from build123d import *

# Parameters (mm, degrees)
F1_DEPTH = 2.54
F4_D     = 6.7564
F5_R     = 5.08
F6_R     = 5.08
F9_D     = 3
F10_D    = 3


with BuildPart() as f1:
    # F0 (on Top) → F1 (new body)
    with BuildSketch(Plane.XY):
        Polygon((-26.9663626849, 16.0324431312), (-26.6666630804, 3.3142461729), (-10.6108812243, 3.3142461729), (-10.6108812243, -5.1539645243), (-26.3746562004, -5.1539645243), (-26.6666630804, -16.9342223267), (-10.6108812243, -17.3322101165), (9.2456126958, -17.3322101165), (9.2456126958, 11.2262545153), (65.6030206382, 11.518263258), (65.6030206382, 16.1625675214), (-11.1902779489, 16.1625675214), align=None)
    extrude(amount=F1_DEPTH)


with BuildPart() as f1_1:
    # F2: moved
    add(f1.part.moved(Location((-33.782, 26.162, 0))))

    # F4 (through all)
    with Locations(Plane.XY.offset(2.54)):
        with Locations((-35.1868793368, 26.1346530169)):
            Hole(F4_D / 2)

    # F5
    f5_edges = [f1_1.edges().sort_by_distance(p)[0] for p in [
        (-60.448663, 9.227778, 1.27),
    ]]
    fillet(f5_edges, radius=F5_R)

    # F6
    f6_edges = [f1_1.edges().sort_by_distance(p)[0] for p in [
        (-60.748363, 42.194443, 1.27),
    ]]
    fillet(f6_edges, radius=F6_R)

    # F9 (through all)
    with Locations(Plane.XY.offset(2.54)):
        with Locations((-52.7054518143, 42.2607827135)):
            Hole(F9_D / 2)

    # F10 (through all)
    with Locations(Plane.XY.offset(2.54)):
        with Locations((-52.9959336795, 9.0430407773)):
            Hole(F10_D / 2)


solid = f1_1.part
Part model, mm, in its own coordinate system. A direction names the side the tool comes from. Coordinates: 2 decimals unless noted, no trailing zeros. Loops run counter-clockwise (first coordinate to the right, second up) from the corner with the lowest first, then second, coordinate; pieces in that order, holes last. Notation, with made-up numbers: (12.25, 4) - (23.25, 4) arc R22 ccw to (23.25, 25) - close; hole circle Ø10 at (-21.5, 87.5). An arc over 180 degrees is marked (long way). Write each question's results on one line, items separated by ' | '. Start each with the question number.
Q1. Which spindle directions (+Z, -Z, +X, -X, +Y, -Y) get a long thin tool onto all of the face, cutting with end or side? Do faces 4 (the flat face through (-6, 42.325, 1)), 5 (the flat face through (-24.536, 23, 1)), 6 (the flat face through (-53, 29.476, 1)). Say none if no direction does.
Q2. Slice it at C-C on y = 11.5. Give the cut face in (x, z), and give its area (3 significant figures).
Q3. Slice it at A-A on z = 1.7. Give the cut face in (x, y), and give its area (3 significant figures).
Q4. Two-plate mould, pull along Y, no slides. Class faces 1 (the flat face through (-44.393, 25, 1)), 2 (the flat face through (-36, 30, 0)), 3 (the flat face through (-35, 8.83, 1)): +Y half, -Y half, draft (parallel to the pull), parting line (faces both ways), or undercut.
Q5. Probe line 1 along X through (y, z) = (26.5, 0.1); line 2 along X through (y, z) = (38.5, 2.3); line 3 along X through (y, z) = (25, 0.8). List the from-to ranges inside material, lowest first.
Q6. Slice it at B-B on x = 8. Give the cut face in (y, z), and give its area (3 significant figures).
Q7. Drop flat-ended pins along their axis: pin 1 Ø1.3 at (x, z) = (-52.5, 1.5) entering from +Y; pin 2 Ø4 at (x, y) = (-35.19, 26.13) entering from -Z; pin 3 Ø1.3 at (y, z) = (25, 1) entering from -X; pin 4 Ø0.8 at (y, z) = (25, 1.5) entering from +X. Give the stop position or say it passes through.
Answer:
1) face 4: +Z, -Z, +X, -X, +Y | face 5: +Z, -Z, +X, -Y | face 6: +Z, -Z, -X
2) outline: (-59.56, 0) - (-24.54, 0) - (-24.54, 2.54) - (-59.56, 2.54) - close | area: 89.0 mm2
3) outline: (-60.63, 37.04) - (-60.45, 29.48) - (-44.39, 29.48) - (-44.39, 21.01) - (-60.16, 21.01) - (-60.32, 14.31) arc R5.08 ccw to (-55.37, 9.1) - (-54.5, 9.08) arc R1.5 cw to (-51.5, 9.01) - (-44.39, 8.83) - (-24.54, 8.83) - (-24.54, 37.39) - (31.82, 37.68) - (31.82, 42.32) - (-44.97, 42.32) - (-51.21, 42.27) arc R1.5 cw to (-54.21, 42.25) - (-55.59, 42.24) arc R5.08 ccw to start; hole circle Ø6.76 at (-35.19, 26.13) | area: 1,280 mm2
4) face 1: undercut | face 2: draft | face 3: -Y half
5) line 1: x = -44.39 to -38.55, -31.83 to -24.54 | line 2: x = -60.45 to 31.82 | line 3: x = -44.39 to -38.37, -32 to -24.54
6) outline: (37.56, 0) - (42.32, 0) - (42.32, 2.54) - (37.56, 2.54) - close | area: 12.1 mm2
7) pin 1: stops at y = 41.03 | pin 2: passes through | pin 3: stops at x = -44.39 | pin 4: stops at x = -24.54
